```python
from build123d import *

# Parameters (mm, degrees)
SKETCH_1_W                  = 100
SKETCH_1_H                  = 160
EXTRUDE_1_DEPTH             = 4
SKETCH_2_R                  = 2
CUT_EXTRUDE_1_DEPTH         = 4
SKETCH_3_R                  = 1.5
CUT_EXTRUDE_2_DEPTH         = 4
SKETCH_4_R                  = 1.5
CUT_EXTRUDE_3_DEPTH         = 4
SKETCH_6_W                  = 100
SKETCH_6_H                  = 4
EXTRUDE_2_DEPTH             = 18
SKETCH_5_R                  = 1.5
CUT_EXTRUDE_4_DEPTH         = 10
PATTERN_LINEAR_1_COUNT      = 2
PATTERN_LINEAR_1_PITCH      = 40
PATTERN_LINEAR_1_COUNT_DIR2 = 2
PATTERN_LINEAR_1_PITCH_DIR2 = 20
MIRROR_3_COPY_1_SKETCH_R    = 1.5
MIRROR_3_COPY_1_DEPTH       = 10
MIRROR_3_COPY_2_SKETCH_R    = 1.5
MIRROR_3_COPY_2_DEPTH       = 10
MIRROR_3_COPY_3_SKETCH_R    = 1.5
MIRROR_3_COPY_3_DEPTH       = 10


with BuildPart() as part:
    # 草图1 → 凸台-拉伸1 (new body)
    with BuildSketch(Plane(origin=(0, 0, 0), x_dir=(1, 0, 0), z_dir=(0, 1, 0))):
        Rectangle(SKETCH_1_W, SKETCH_1_H)
    extrude(amount=EXTRUDE_1_DEPTH)

    # 草图2 → 切除-拉伸1 (cut)
    with BuildSketch(Plane(origin=(0, 4, 0), x_dir=(1, 0, 0), z_dir=(0, 1, 0))):
        with Locations(Location((40, -3, 0), (0, 0, 270))):
            Circle(SKETCH_2_R)
        with Locations(Location((26, -3, 0), (0, 0, 270))):
            Circle(SKETCH_2_R)
        with Locations(Location((40, -35, 0), (0, 0, 90))):
            Circle(SKETCH_2_R)
        with Locations(Location((26, -35, 0), (0, 0, 90))):
            Circle(SKETCH_2_R)
    extrude(amount=-CUT_EXTRUDE_1_DEPTH, mode=Mode.SUBTRACT)

    # 草图3 → 切除-拉伸2 (cut)
    with BuildSketch(Plane(origin=(0, 4, 0), x_dir=(1, 0, 0), z_dir=(0, 1, 0))):
        with Locations(Location((-39, 44, 0), (0, 0, 270))):
            Circle(SKETCH_3_R)
        with Locations(Location((-11, 44, 0), (0, 0, 270))):
            Circle(SKETCH_3_R)
        with Locations(Location((-11, 16, 0), (0, 0, 270))):
            Circle(SKETCH_3_R)
        with Locations(Location((-39, 16, 0), (0, 0, 270))):
            Circle(SKETCH_3_R)
    cut_extrude_2 = extrude(amount=-CUT_EXTRUDE_2_DEPTH, mode=Mode.SUBTRACT)

    # 镜向1: 切除-拉伸2 across plane
    add(cut_extrude_2.mirror(Plane.XY), mode=Mode.SUBTRACT)

    # 草图4 → 切除-拉伸3 (cut)
    with BuildSketch(Plane(origin=(0, 4, 0), x_dir=(1, 0, 0), z_dir=(0, 1, 0))):
        with Locations(Location((42, 12, 0), (0, 0, 270))):
            Circle(SKETCH_4_R)
        with Locations(Location((8, 12, 0), (0, 0, 90))):
            Circle(SKETCH_4_R)
        with Locations(Location((42, -12, 0), (0, 0, 90))):
            Circle(SKETCH_4_R)
        with Locations(Location((8, -12, 0), (0, 0, 270))):
            Circle(SKETCH_4_R)
    extrude(amount=-CUT_EXTRUDE_3_DEPTH, mode=Mode.SUBTRACT)

    # 草图6 → 凸台-拉伸2 (add)
    with BuildSketch(Plane(origin=(0, 0, -80), x_dir=(-1, 0, 0), z_dir=(0, 0, -1))):
        with Locations((0, 2)):
            Rectangle(SKETCH_6_W, SKETCH_6_H)
    extrude_2 = extrude(amount=EXTRUDE_2_DEPTH)

    # 草图5 → 切除-拉伸4 (cut)
    with BuildSketch(Plane(origin=(0, 4, 0), x_dir=(1, 0, 0), z_dir=(0, 1, 0))):
        with Locations(Location((-35, 93, 0), (0, 0, 270))):
            Circle(SKETCH_5_R)
    cut_extrude_4 = extrude(amount=-CUT_EXTRUDE_4_DEPTH, mode=Mode.SUBTRACT)

    # 镜向2: 凸台-拉伸2 across plane
    add(extrude_2.mirror(Plane.XY))

    # 阵列(线性)1: Cut-Extrude 4 2 × 2
    with Locations(*[(j * PATTERN_LINEAR_1_PITCH_DIR2, 0, i * PATTERN_LINEAR_1_PITCH) for i in range(PATTERN_LINEAR_1_COUNT) for j in range(PATTERN_LINEAR_1_COUNT_DIR2) if (i, j) != (0, 0)]):
        add(cut_extrude_4, mode=Mode.SUBTRACT)

    # 镜向3: 切除-拉伸4 across plane
    add(cut_extrude_4.mirror(Plane.XY), mode=Mode.SUBTRACT)

    # 镜向3 copy 1 sketch → 镜向3 copy 1 (cut)
    with BuildSketch(Plane(origin=(20, 4, 0), x_dir=(1, 0, 0), z_dir=(0, 1, 0))):
        with Locations((-35, -93)):
            Circle(MIRROR_3_COPY_1_SKETCH_R)
    extrude(amount=-MIRROR_3_COPY_1_DEPTH, mode=Mode.SUBTRACT)

    # 镜向3 copy 2 sketch → 镜向3 copy 2 (cut)
    with BuildSketch(Plane(origin=(0, 4, -40), x_dir=(1, 0, 0), z_dir=(0, 1, 0))):
        with Locations((-35, -93)):
            Circle(MIRROR_3_COPY_2_SKETCH_R)
    extrude(amount=-MIRROR_3_COPY_2_DEPTH, mode=Mode.SUBTRACT)

    # 镜向3 copy 3 sketch → 镜向3 copy 3 (cut)
    with BuildSketch(Plane(origin=(20, 4, -40), x_dir=(1, 0, 0), z_dir=(0, 1, 0))):
        with Locations((-35, -93)):
            Circle(MIRROR_3_COPY_3_SKETCH_R)
    extrude(amount=-MIRROR_3_COPY_3_DEPTH, mode=Mode.SUBTRACT)


solid = part.part
```
Verification items for the finished model (mm, model axes). Give positions to 0.01 mm unless a question says otherwise; leave off trailing zeros. Loops run counter-clockwise (first coordinate to the right, second up) from the corner with the lowest first, then second, coordinate; pieces in that order, holes last.
1. Thickness scan on line 1 (X direction, y = 0.95, z = -93); line 2 (X direction, y = 3.25, z = -44); line 3 (Z direction, x = 39, y = 3.65). Record the ranges inside material, lowest first.
2. Section check A-A, the plane x = 26. Enter the section's corners in (y, z), then the cut area to 3 significant figures.
3. Mould release check, pull along Z, two halves, no side actions. Record for faces 1 (the flat face through (1, 2, -98)), 2 (the cylindrical face through (38, 2, 3)), 3 (the flat face through (1, 4, -1)): released by +Z, released by -Z, zero draft, split by the parting line, or undercut.
Geometry says:
1. line 1: x = -50 to -36.5, -33.5 to -16.5, -13.5 to 50
1. line 2: x = -50 to -40.5, -37.5 to -12.5, -9.5 to 50
1. line 3: z = -98 to 1.27, 4.73 to 33.27, 36.73 to 98
2. outline: (0, -98) - (4, -98) - (4, 1) - (0, 1) - close; (0, 5) - (4, 5) - (4, 33) - (0, 33) - close; (0, 37) - (4, 37) - (4, 98) - (0, 98) - close
2. area: 752 mm2
3. face 1: released by -Z
3. face 2: undercut
3. face 3: zero draft
